Can you work these out from the model? Positions are in its coordinate system, mm. Round coordinates to 2 decimals unless told otherwise and drop trailing zeros. Loops run counter-clockwise (first coordinate to the right, second up) from the corner with the lowest first, then second, coordinate; pieces in that order, holes last. Notation, with made-up numbers: M -11.75,-27.5 L 10.25,-27.5 A20 cw 10.25,4.5 Z; hole C 19,-19.75 d8. An arc over 180 degrees is marked long. Answer as CSV lines item,"result".
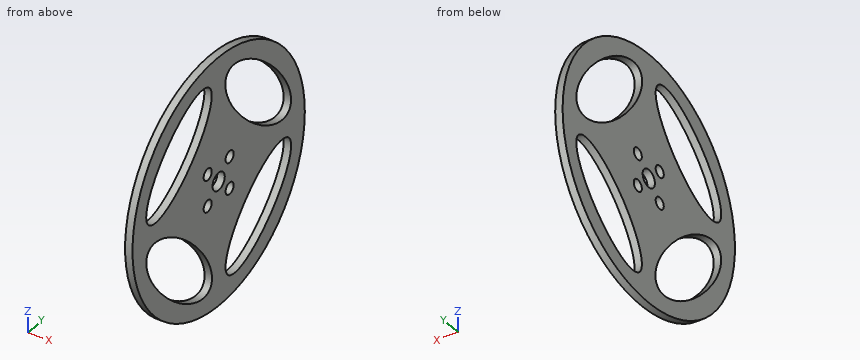
from build123d import *

# Parameters (mm, degrees)
SKIZZE1_W                        = 3
SKIZZE1_H                        = 46.45
F_4_7_4_7_DURCHMESSER_BOHRUNG1_D = 4.7
SKIZZE5_RX                       = 25
SKIZZE5_RY                       = 10
SCHNITT_LINEAR_AUSTRAGEN1_DEPTH  = 3
KREISMUSTER1_COUNT               = 4


with BuildPart() as part:
    # Skizze1 → Rotation1 (revolve)
    with BuildSketch(Plane.XY):
        with Locations((-39.553372853, 36.525)):
            Rectangle(SKIZZE1_W, SKIZZE1_H)
    revolve(axis=Axis((-17.6629112, 9.75, 0), (-1, 0, 0)))

    # Ø4.7 (4.7) Durchmesser Bohrung1 (through all)
    with Locations(Plane(origin=(-41.053372853, 11.968723204, 19.868936148), x_dir=(0, 0, 1), z_dir=(-1, 0, 0))):
        with Locations((-13.504975118, -8.582684234), (-26.232897179, -8.582684234), (-26.232897179, 4.145237827), (-13.504975118, 4.145237827)):
            Hole(F_4_7_4_7_DURCHMESSER_BOHRUNG1_D / 2)

    # Skizze5 → Schnitt-Linear austragen1 (cut)
    with BuildSketch(Plane(origin=(-38.053372853, 0, 0), x_dir=(0, 0, -1), z_dir=(1, 0, 0))):
        with Locations(Location((-23.027329597, 32.684515508), (0, 0, 45.090609512))):
            Ellipse(SKIZZE5_RX, SKIZZE5_RY)
    schnitt_linear_austragen1 = extrude(amount=-SCHNITT_LINEAR_AUSTRAGEN1_DEPTH, mode=Mode.SUBTRACT)

    # Kreismuster1: Schnitt-Linear austragen1 ×4 about axis
    kreismuster1_axis = Axis((0, 9.75, 0), (-1, 0, 0))
    for i in range(1, KREISMUSTER1_COUNT):
        add(schnitt_linear_austragen1.rotate(kreismuster1_axis, i * 360 / KREISMUSTER1_COUNT), mode=Mode.SUBTRACT)


solid = part.part
Item 1: If we section it at B-B on y = 9.75: Write out the boundary of the cut face in (x, z), then the cut area to 3 significant figures.
Output:
outline,"M -41.05,-50 L -38.05,-50 L -38.05,-3.55 L -41.05,-3.55 Z; M -41.05,3.55 L -38.05,3.55 L -38.05,50 L -41.05,50 Z"
area,"279 mm2"
Item 2: If we section it at A-A on z = 0: Write out the boundary of the cut face in (x, y), then the cut area to 3 significant figures.
Output:
outline,"M -41.05,-40.25 L -38.05,-40.25 L -38.05,6.2 L -41.05,6.2 Z; M -41.05,13.3 L -38.05,13.3 L -38.05,59.75 L -41.05,59.75 Z"
area,"279 mm2"
Item 3: Will these pins go through, and if not, where does the flat tip stop? pin 1 (1 mm diameter, centred on x = -38.5, y = 22, fed in from -Z); pin 2 (4.5 mm diameter, centred on y = 9.75, z = 0, fed in from -X); pin 3 (10 mm diameter, centred on y = 39, z = 10.5, fed in from +X); pin 4 (1.5 mm diameter, centred on x = -40.5, z = 9, fed in from -Y).
Output:
pin 1,"stops at z = -48.6"
pin 2,"passes through"
pin 3,"stops at x = -38.05"
pin 4,"stops at y = -39.56"
Item 4: If we section it at C-C on y = 38.5: State how many separate pieces and enclosed holes the cut face has, then the cut area to 3 significant figures.
Output:
separate pieces,"3"
enclosed holes,"0"
area,"95.3 mm2"
Item 5: If I drill on line 1 along Y through (x, z) = (-39.05, 0); line 2 along Z through (x, y) = (-39.6, -15.5); line 3 along Z through (x, y) = (-39.95, -23.5), over which ranges is the centre line in solid material (lowest first)? Write a range as from..to.
Output:
line 1,"y = -40.25..6.2, 13.3..59.75"
line 2,"z = -43.16..-34.37, -8.34..8.27, 34.38..43.16"
line 3,"z = -37.34..-26.6, -4.55..4.43, 26.6..37.34"
